Input: part model. Units: mm. Frame: model coordinates. Coordinates: 2 decimals unless noted, no trailing zeros. Loops run counter-clockwise (first coordinate to the right, second up) from the corner with the lowest first, then second, coordinate; pieces in that order, holes last.
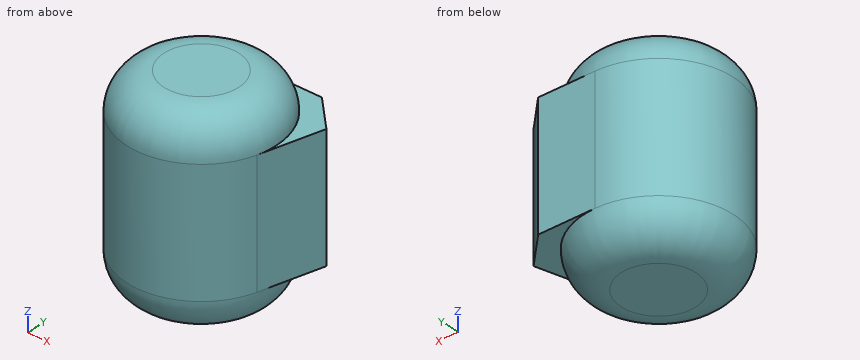
```python
from build123d import *

# Parameters (mm, degrees)
F0_R     = 300
F1_DEPTH = 800
F2_R     = 150
F4_START = -150
F4_DEPTH = 500


with BuildPart() as f1:
    # F0 (on Top) → F1 (new body)
    with BuildSketch(Plane.XY):
        Circle(F0_R)
    extrude(amount=F1_DEPTH)

    # F2
    f2_edges = [f1.edges().sort_by_distance(p)[0] for p in [
        (-300, 0, 800),
        (-300, 0, 0),
    ]]
    fillet(f2_edges, radius=F2_R)

    # F3 (on face) → F4 (join)
    with BuildSketch(Plane.XY.offset(800).offset(F4_START)):
        with BuildLine():
            Line((229.2893218813, 300), (0, 300))
            ThreePointArc((0, 300), (114.8050297095, 277.1638597534), (212.132034356, 212.132034356))
            Line((212.132034356, 212.132034356), (264.6446609407, 264.6446609407))
            Line((264.6446609407, 264.6446609407), (229.2893218813, 300))
        make_face()
        with BuildLine():
            ThreePointArc((212.132034356, 212.132034356), (277.1638597534, 114.8050297095), (300, 0))
            Line((300, 0), (300, 229.2893218813))
            Line((300, 229.2893218813), (264.6446609407, 264.6446609407))
            Line((264.6446609407, 264.6446609407), (212.132034356, 212.132034356))
        make_face()
        with BuildLine():
            Line((300, 229.2893218813), (300, 0))
            ThreePointArc((300, 0), (297.5110648624, -38.5637949955), (290.0855581037, -76.4877047615))
            Line((290.0855581037, -76.4877047615), (355.9564720177, 173.3328498637))
            Line((355.9564720177, 173.3328498637), (300, 229.2893218813))
        make_face()
    extrude(amount=-F4_DEPTH)


solid = f1.part
```
Item 1: Section query A-A (z = 160.5). Output: boundary loops of the cut face in (x, y), then the cut area to 3 significant figures.
Result:
outline: (0, 300) arc R300 ccw (long way) to (290.09, -76.49) - (355.96, 173.33) - (229.29, 300) - close
area: 307,000 mm2
Item 2: Line query: L1, parallel to Z at x = 176.5, y = -206.5; L2, parallel to X at y = 215.5, z = 71; L3, parallel to Z at x = -189, y = -28. Output: solid intervals per line, ascending.
Result:
L1: z = 62.25 to 737.75
L2: x = -174.85 to 174.85
L3: z = 5.73 to 794.27
Item 3: Contact query for flat-ended pins moving along their axis: P1, Ø6, axis at x = -155, y = 206.5, coming from the -Z side (3 decimals); P2, Ø12, axis at y = 166, z = 254, coming from the +X side; P3, Ø1.5, axis at x = 235.5, y = 151, coming from the +Z side. Output: stop coordinate, or through.
Result:
P1: stops at z = 43.075
P2: stops at x = 355.61
P3: stops at z = 726.54
